Check sheet for the modelled part. Datum: model origin and axes. Units: mm. Face numbers are marked on the shaded views. A direction names the side the tool comes from. Round coordinates to 2 decimals unless told otherwise and drop trailing zeros. Order: outer loops, then holes, each group sorted by start corner. A loop starts at its lowest first (then second) coordinate and runs counter-clockwise, first axis right, second up.
```python
from build123d import *

# Parameters (mm, degrees)
SKETCH2_R      = 1.275
SHAFT_DEPTH    = 40.4
SKETCH5_R      = 2.725
HEAD_DEPTH     = 3
CHAMFER1_SIZE  = 0.25
CHAMFER1_SIZE2 = 0.357037002
DEBURS_SIZE    = 0.2


with BuildPart() as part:
    # Sketch2 → Shaft (new body)
    with BuildSketch(Plane.XY):
        Circle(SKETCH2_R)
    extrude(amount=SHAFT_DEPTH)

    # Sketch5 → Head (add)
    with BuildSketch(Plane.XY):
        Circle(SKETCH5_R)
    extrude(amount=-HEAD_DEPTH)

    # Chamfer1
    chamfer1_edges = [part.edges().sort_by_distance(p)[0] for p in [
        (-1.275, 0, 40.4),
    ]]
    chamfer1_side = [part.faces().sort_by_distance(p)[0] for p in [
        (0, 0, 40.4),
    ]]
    chamfer(chamfer1_edges, length=CHAMFER1_SIZE, length2=CHAMFER1_SIZE2, reference=chamfer1_side[0])

    # Deburs
    deburs_edges = [part.edges().sort_by_distance(p)[0] for p in [
        (-2.725, 0, -3),
        (-2.725, 0, 0),
    ]]
    chamfer(deburs_edges, length=DEBURS_SIZE)

    # Sketch6 → e-Clip Notch Long (revolve, cut)
    with BuildSketch(Plane(origin=(0, 0, 0), x_dir=(0, 0, -1), z_dir=(1, 0, 0))):
        Polygon((-39.4, 1.275), (-38.4, 1.275), (-38.8, 0.875), (-39, 0.875), align=None)
    revolve(axis=Axis((0, 0, 0), (0, 0, 1)), mode=Mode.SUBTRACT)


solid = part.part
```
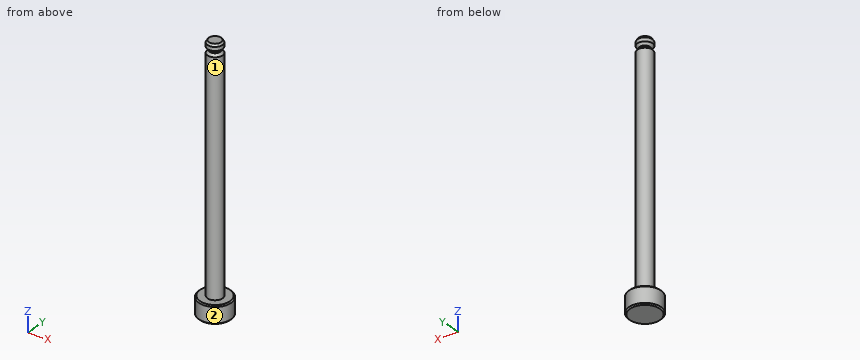
Item 1: Access from +Z, -Z, +X, -X, +Y, -Y to the whole of each face (thin tool, end or side, straight path). Record for the marked faces 1 and 2.
Answer:
face 1: +Z
face 2: +Z, -Z
Item 2: Scan lines: line 1 along Z through (x, y) = (0.55, -2.45); line 2 along X through (y, z) = (0.15, 22). Record each from-to range of solid material in increasing order.
Answer:
line 1: z = -3 to 0
line 2: x = -1.27 to 1.27
Item 3: Go/stop test with flat-tipped pins: P1, Ø3, axis at x = 1, z = 4, coming from the -Y side (3 decimals); P2, Ø1.5, axis at y = 1, z = 29, coming from the +X side; P3, Ø1.5, axis at y = 0, z = 10, coming from the -X side (3 decimals). Record where each tip stops, or that it passes through.
Answer:
P1: stops at y = -1.275
P2: stops at x = 1.25
P3: stops at x = -1.275
Item 4: Sectioned sample at A-A (y = 0). Record the cut outline in (x, z) (3 decimals).
Answer:
outline: (-2.725, -2.8) - (-2.525, -3) - (2.525, -3) - (2.725, -2.8) - (2.725, -0.2) - (2.525, 0) - (1.275, 0) - (1.275, 38.4) - (0.875, 38.8) - (0.875, 39) - (1.275, 39.4) - (1.275, 40.043) - (1.025, 40.4) - (-1.025, 40.4) - (-1.275, 40.043) - (-1.275, 39.4) - (-0.875, 39) - (-0.875, 38.8) - (-1.275, 38.4) - (-1.275, 0) - (-2.525, 0) - (-2.725, -0.2) - close
Item 5: Sectioned sample at C-C (z = 28). Record the cut outline in (x, y) (3 decimals), and give its area (3 significant figures).
Answer:
outline: circle Ø2.55 at (0, 0)
area: 5.11 mm2
